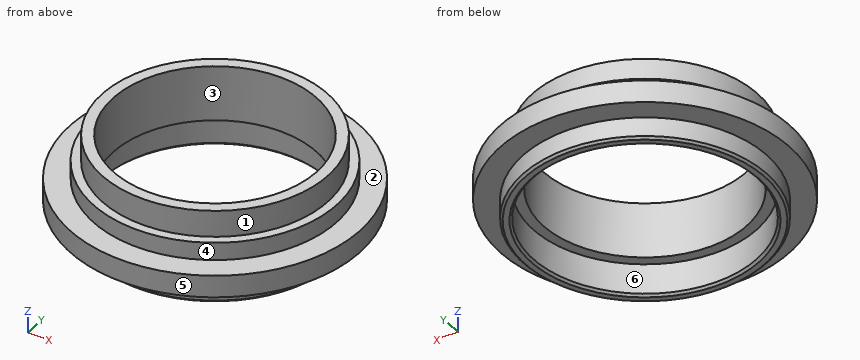
from build123d import *

# Parameters (mm, degrees)
CHAMFER1_SIZE = 0.5


with BuildPart() as part:
    # Sketch1 → Revolve1 (revolve)
    with BuildSketch(Plane(origin=(0, 0, 0), x_dir=(1, 0, 0), z_dir=(0, 1, 0)), mode=Mode.PRIVATE) as revolve1_sk:
        Polygon((25.3, 19.8), (27.6, 19.8), (27.6, 15), (32.75, 15), (32.75, 10), (27.5, 10), (27.5, 6), (25.5, 6), (25.5, 0), (23, 0), (23, 12.5), (25.3, 12.5), align=None)
    revolve(revolve1_sk.sketch.rotate(Axis((0, 0, -99.297916667), (0, 0, 1)), 180), axis=Axis((0, 0, -99.297916667), (0, 0, 1)))

    # Chamfer1
    chamfer1_edges = [part.edges().sort_by_distance(p)[0] for p in [
        (27.6, 0, -19.8),
        (25.3, 0, -19.8),
    ]]
    chamfer(chamfer1_edges, length=CHAMFER1_SIZE)


solid = part.part
For this review, take the finished solid that the model builds, in its own axes (mm). Face numbers are marked on the shaded views. A direction names the side the tool comes from. Give positions to 0.01 mm unless a question says otherwise; leave off trailing zeros. Loops run counter-clockwise (first coordinate to the right, second up) from the corner with the lowest first, then second, coordinate; pieces in that order, holes last.
Item 1: Tool access review of the marked faces 4, 5 and 6: name each direction out of +Z, -Z, +X, -X, +Y, -Y from which nothing blocks a thin tool from reaching the whole face with its end or side.
Item 2: Take a section at A-A, the plane y = 0. State the section outline as (x, z) points.
Item 3: For line 1 along Y through (x, z) = (0, -18); line 2 along Y through (x, z) = (0, -14.75); line 3 along Z through (x, y) = (12.5, -21), list the stretches that pass through material, from the lowest coordinate up.
Item 4: Insertion check: pin 1 (8 mm diameter, centred on x = -12, y = 23, fed in from +Z); pin 2 (2 mm diameter, centred on y = -11, z = -8, fed in from -X); pin 3 (6 mm diameter, centred on y = 19.5, z = -10, fed in from -X); pin 4 (2 mm diameter, centred on x = -1.5, z = -6, fed in from -Y). Each pin has a flat end and moves straight along its axis. Give the tip position at first contact, or say it passes through.
Item 5: Draft analysis for pull direction Y (two halves, no side actions). For the marked faces 1, 2 and 3, state which applies: +Y half, -Y half, draft (parallel to the pull), parting line (faces both ways), or undercut.
Item 6: Take a section at C-C, the plane z = -3.25. State the section outline as (x, y) points, and give its area (3 significant figures).
Calculated:
1. face 4: +Z
1. face 5: +Z, -Z
1. face 6: -Z
2. outline: (-32.75, -15) - (-27.6, -15) - (-27.6, -19.3) - (-27.1, -19.8) - (-25.8, -19.8) - (-25.3, -19.3) - (-25.3, -12.5) - (-23, -12.5) - (-23, 0) - (-25.5, 0) - (-25.5, -6) - (-27.5, -6) - (-27.5, -10) - (-32.75, -10) - close; (23, -12.5) - (25.3, -12.5) - (25.3, -19.3) - (25.8, -19.8) - (27.1, -19.8) - (27.6, -19.3) - (27.6, -15) - (32.75, -15) - (32.75, -10) - (27.5, -10) - (27.5, -6) - (25.5, -6) - (25.5, 0) - (23, 0) - close
3. line 1: y = -27.6 to -25.3, 25.3 to 27.6
3. line 2: y = -32.75 to -25.3, 25.3 to 32.75
3. line 3: z = -12.5 to 0
4. pin 1: stops at z = 0
4. pin 2: stops at x = -25.62
4. pin 3: stops at x = -28.29
4. pin 4: stops at y = -27.5
5. face 1: parting line
5. face 2: draft
5. face 3: undercut
6. outline: circle Ø51 at (0, 0); hole circle Ø46 at (0, 0)
6. area: 381 mm2
